from build123d import *

# Parameters (mm, degrees)
F1_DEPTH = 12.7
F0_R     = 31.61033
F2_DEPTH = 43.18
F4_DEPTH = 6.35


with BuildPart() as f1:
    # F0 (on Top) → F1 (new body)
    with BuildSketch(Plane.XY):
        with BuildLine():
            Line((-32.126933, 27.557764), (-107.518122, 27.557764))
            Line((-107.518122, 27.557764), (-107.518122, -27.557764))
            Line((-107.518122, -27.557764), (-32.126933, -27.557764))
            Line((-32.126933, -27.557764), (-32.126933, -27.209316))
            ThreePointArc((-32.126933, -27.209316), (-42.100911, 0), (-32.126933, 27.209316))
            Line((-32.126933, 27.209316), (-32.126933, 27.557764))
        make_face()
    extrude(amount=F1_DEPTH)

    # F0 (on Top) → F2 (join)
    with BuildSketch(Plane.XY):
        with BuildLine():
            ThreePointArc((42.100911, 0), (14.489886, 39.52885), (-32.126933, 27.209316))
            ThreePointArc((-32.126933, 27.209316), (-42.100911, 0), (-32.126933, -27.209316))
            ThreePointArc((-32.126933, -27.209316), (14.489886, -39.52885), (42.100911, 0))
        make_face()
        Circle(F0_R, mode=Mode.SUBTRACT)
    extrude(amount=F2_DEPTH)

    # F3 (on Front) → F4 (join, symmetric)
    with BuildSketch(Plane.XZ):
        Polygon((-41.93845, 10.919823), (-41.93845, 37.190702), (-73.273592, 10.919823), align=None)
    extrude(amount=F4_DEPTH, both=True)


solid = f1.part
Can you work these out from the model? Positions are in its coordinate system, mm. A direction names the side the tool comes from. Coordinates: 2 decimals unless noted, no trailing zeros. Order: outer loops, then holes, each group sorted by start corner. A loop starts at its lowest first (then second) coordinate and runs counter-clockwise, first axis right, second up. Notation, with made-up numbers: (4, 61) -> (31, 61) arc R18 cw to (31, 70) -> close; hole circle Ø2 at (42.5, 37). An arc over 180 degrees is marked (long way). Use one line per item in the form item = value.
Q1. Imagine slicing it at C-C, the plane y = -16.5. List the corners of the cut face in (x, z) for me, then the cut area to 3 significant figures.
From the geometry:
outline = (-107.52, 0) -> (-26.96, 0) -> (-26.96, 43.18) -> (-38.73, 43.18) -> (-38.73, 12.7) -> (-107.52, 12.7) -> close; (26.96, 0) -> (38.73, 0) -> (38.73, 43.18) -> (26.96, 43.18) -> close
area = 1,890 mm²
Q2. Imagine slicing it at D-D, the plane y = 13.5. List the corners of the cut face in (x, z) for me.
From the geometry:
outline = (-107.52, 0) -> (-28.58, 0) -> (-28.58, 43.18) -> (-39.88, 43.18) -> (-39.88, 12.7) -> (-107.52, 12.7) -> close; (28.58, 0) -> (39.88, 0) -> (39.88, 43.18) -> (28.58, 43.18) -> close
Q3. I need wall thicknesses on L1, parallel to Y at x = 0, z = 12; L2, parallel to Y at x = -7, z = 7; L3, parallel to X at y = -19.5, z = 39.5. Which ranges of each line are inside material? Lowest first, please.
From the geometry:
L1 = -42.1 to -31.61, 31.61 to 42.1
L2 = -41.51 to -30.83, 30.83 to 41.51
L3 = -37.31 to -24.88, 24.88 to 37.31
Q4. Imagine slicing it at A-A, the plane z = 7. List the corners of the cut face in (x, y) for me.
From the geometry:
outline = (-107.52, -27.56) -> (-32.13, -27.56) -> (-32.13, -27.21) arc R42.1 ccw to (42.1, 0) arc R42.1 ccw to (-32.13, 27.21) -> (-32.13, 27.56) -> (-107.52, 27.56) -> close; hole circle Ø63.22 at (0, 0)
Q5. Will these pins go through, and if not, where does the flat tip stop? P1, Ø1, axis at x = -18, z = 21.5, coming from the -Y side; P2, Ø3, axis at y = -20, z = 29.5, coming from the +X side; P3, Ø6.5, axis at x = -51, z = 3.5, coming from the -Y side.
From the geometry:
P1 = -38.29
P2 = 37.82
P3 = -27.56
Q6. Imagine slicing it at B-B, the plane x = 0. List the corners of the cut face in (y, z) for me, then the cut area to 3 significant figures.
From the geometry:
outline = (-42.1, 0) -> (-31.61, 0) -> (-31.61, 43.18) -> (-42.1, 43.18) -> close; (31.61, 0) -> (42.1, 0) -> (42.1, 43.18) -> (31.61, 43.18) -> close
area = 906 mm²
Q7. We'd pull the mould along X, two halves only. Please class faces 4 (the face through (-56.34, -0.089, 25.117)), 5 (the face through (-50, 6.35, 20)), 6 (the face through (-4.12, 31.34, 21.29)): released by +X, released by -X, zero draft, split by the parting line, or undercut.
From the geometry:
face_4 = released by -X
face_5 = zero draft
face_6 = undercut
Q8. Which directions (+Z, -Z, +X, -X, +Y, -Y) give clear straight access to the entire face, cutting with the end or side of a thin tool? Please do faces 1 (the face through (-70, -27.558, 6)), 2 (the face through (-69, 27.558, 6)), 3 (the face through (-50, -6.35, 20)).
From the geometry:
face_1 = +Z, -Z, -X, -Y
face_2 = +Z, -Z, -X, +Y
face_3 = +Z, -X, -Y
